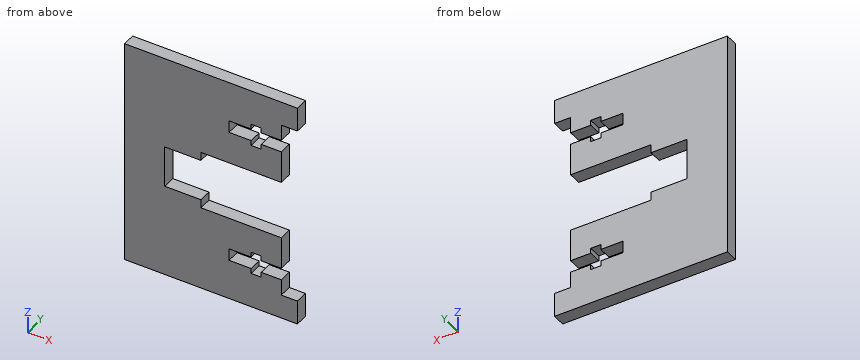
Autodesk Inventor part; units mm, degrees
ref_plane "YZ Plane" through (0, 0, 0) normal (1, 0, 0) x (0, 1, 0)
ref_plane "XZ Plane" through (0, 0, 0) normal (0, 1, 0) x (-1, 0, 0)
ref_plane "XY Plane" through (0, 0, 0) normal (0, 0, 1) x (1, 0, 0)
sketch "Sketch1" plane through (0, 0, 0) normal (0, 1, 0) x (-1, 0, 0)
  line L0 (38.3151, 0) -> (38.3151, -28.25)
  line L1 (38.3151, -28.25) -> (-4.6849, -28.25)
  line L2 (-4.6849, -28.25) -> (-4.6849, -22.25)
  line L3 (-4.6849, -22.25) -> (-0.6849, -22.25)
  line L4 (-0.6849, -22.25) -> (-0.6849, -18.25)
  line L5 (-0.6849, -18.25) -> (4.3151, -18.25)
  line L6 (4.3151, -18.25) -> (4.3151, -19.525)
  line L7 (4.3151, -19.525) -> (6.8151, -19.525)
  line L8 (6.8151, -13.975) -> (4.3151, -13.975)
  line L9 (4.3151, -13.975) -> (4.3151, -15.25)
  line L10 (4.3151, -15.25) -> (-0.6849, -15.25)
  line L11 (-0.6849, -15.25) -> (-0.6849, -7.25)
  line L12 (-0.6849, -7.25) -> (19.3151, -7.25)
  line L13 (19.3151, -7.25) -> (19.3151, -5.15)
  line L14 (19.3151, -5.15) -> (28.3151, -5.15)
  line L15 (28.3151, -5.15) -> (28.3151, 0)
  line L16 (0, 0) -> (38.3151, 0) construction
  line L17 (6.8151, -15.25) -> (12.3151, -15.25)
  line L18 (12.3151, -15.25) -> (12.3151, -18.25)
  line L19 (12.3151, -18.25) -> (6.8151, -18.25)
  line L20 (6.8151, -19.525) -> (6.8151, -18.25)
  line L21 (6.8151, -15.25) -> (6.8151, -13.975)
  line L22 (38.3151, 0) -> (38.3151, 28.25)
  line L23 (38.3151, 28.25) -> (-4.6849, 28.25)
  line L24 (-4.6849, 28.25) -> (-4.6849, 22.25)
  line L25 (-4.6849, 22.25) -> (-0.6849, 22.25)
  line L26 (-0.6849, 22.25) -> (-0.6849, 18.25)
  line L27 (-0.6849, 18.25) -> (4.3151, 18.25)
  line L28 (4.3151, 18.25) -> (4.3151, 19.525)
  line L29 (4.3151, 19.525) -> (6.8151, 19.525)
  line L30 (6.8151, 13.975) -> (4.3151, 13.975)
  line L31 (4.3151, 13.975) -> (4.3151, 15.25)
  line L32 (4.3151, 15.25) -> (-0.6849, 15.25)
  line L33 (-0.6849, 15.25) -> (-0.6849, 7.25)
  line L34 (-0.6849, 7.25) -> (19.3151, 7.25)
  line L35 (19.3151, 7.25) -> (19.3151, 5.15)
  line L36 (19.3151, 5.15) -> (28.3151, 5.15)
  line L37 (28.3151, 5.15) -> (28.3151, 0)
  line L38 (6.8151, 15.25) -> (12.3151, 15.25)
  line L39 (12.3151, 15.25) -> (12.3151, 18.25)
  line L40 (12.3151, 18.25) -> (6.8151, 18.25)
  line L41 (6.8151, 19.525) -> (6.8151, 18.25)
  line L42 (6.8151, 15.25) -> (6.8151, 13.975)
  dimension "d0" = 5.55
  dimension "d1" = 2.5
  dimension "d2" = 3
  dimension "d3" = 6
  dimension "d4" = 5
  dimension "d7" = 4
  dimension "d9" = 24
  dimension "d10" = 17
  dimension "d11" = 10.3
  dimension "d12" = 9
  dimension "d13" = 14.5
  dimension "d14" = 8
  dimension "d15" = 4
  dimension "d16" = 10
extrude "Extrusion1" add sketch "Sketch1" along normal blind 3.2
properties part number "Soporte_Plug_Alimentacion"
Part model, mm, in its own coordinate system. Round coordinates to 2 decimals unless told otherwise and drop trailing zeros. Write each loop counter-clockwise with the first axis right and the second up, starting at its lowest first coordinate (ties: lowest second). Pieces come first, ordered by that corner, then holes. Notation, with made-up numbers: (32, 18) -> (66, 18) arc R26 ccw to (66, 35) -> close; hole circle Ø2 at (37, 67.5). An arc over 180 degrees is marked (long way). Return JSON: item names as keys, results as strings. Group by question number.
Q1. Saw through at D-D on x = -16. Write the cut outline in (y, z), plus the area to 3 significant figures.
Q2. Saw through at B-B on x = -26.5. Write the cut outline in (y, z), plus the area to 3 significant figures.
Q3. Saw through at C-C on z = 6.5. Write the cut outline in (x, y), plus the area to 3 significant figures.
Q4. Saw through at A-A on x = -7.5. Write the cut outline in (y, z).
Q5. Probe L1, parallel to Z at x = -6, y = 0.6 (3 decimals); L2, parallel to Z at x = 1.5, y = 2.6; L3, parallel to Z at x = -0.5, y = 3.05. List the from-to ranges inside material, lowest first. Write a range as [from, to].
Q6. Pin check, flat tips, straight feed: pin 1 (0.6 mm diameter, centred on y = 2.5, z = -6, fed in from +X); pin 2 (1.7 mm diameter, centred on y = 2.5, z = 6.5, fed in from +X). Stop position of each tip, or through.
Answer:
{
 "1": {"outline": "(0, -28.25) -> (3.2, -28.25) -> (3.2, -7.25) -> (0, -7.25) -> close; (0, 7.25) -> (3.2, 7.25) -> (3.2, 28.25) -> (0, 28.25) -> close", "area": "134 mm2"},
 "2": {"outline": "(0, -28.25) -> (3.2, -28.25) -> (3.2, -5.15) -> (0, -5.15) -> close; (0, 5.15) -> (3.2, 5.15) -> (3.2, 28.25) -> (0, 28.25) -> close", "area": "148 mm2"},
 "3": {"outline": "(-38.32, 0) -> (-19.32, 0) -> (-19.32, 3.2) -> (-38.32, 3.2) -> close", "area": "60.8 mm2"},
 "4": {"outline": "(0, -28.25) -> (3.2, -28.25) -> (3.2, -18.25) -> (0, -18.25) -> close; (0, -15.25) -> (3.2, -15.25) -> (3.2, -7.25) -> (0, -7.25) -> close; (0, 7.25) -> (3.2, 7.25) -> (3.2, 15.25) -> (0, 15.25) -> close; (0, 18.25) -> (3.2, 18.25) -> (3.2, 28.25) -> (0, 28.25) -> close"},
 "5": {"L1": "[-28.25, -19.525], [-13.975, -7.25], [7.25, 13.975], [19.525, 28.25]", "L2": "[-28.25, -22.25], [22.25, 28.25]", "L3": "[-28.25, -18.25], [-15.25, -7.25], [7.25, 15.25], [18.25, 28.25]"},
 "6": {"pin 1": "x = -19.32", "pin 2": "x = 0.68"}
}
